The model under review builds one solid part; all positions refer to its coordinate system, in mm. A direction names the side the tool comes from. Round coordinates to 2 decimals unless told otherwise and drop trailing zeros. Order: outer loops, then holes, each group sorted by start corner. A loop starts at its lowest first (then second) coordinate and runs counter-clockwise, first axis right, second up. Notation, with made-up numbers: M 13,57 L 23,57 A12 cw 23,69 Z; hole C 39,-30 d8. An arc over 180 degrees is marked long. Answer as a JSON object with one key per item and string values. Group by question number.
1. To check wall thickness, follow probe 1 along X at (y, z) = (5, 33); probe 2 along X at (y, z) = (7.5, 24.5); probe 3 along X at (y, z) = (-6.5, 54.5). State the ranges of each line that lie inside material, in increasing order. Write a range as [from, to].
2. Add section A-A on y = -5. State the section outline as (x, z) points.
3. Add section B-B on y = 15.5. State the section outline as (x, z) points.
4. Add section C-C on x = 26. State the section outline as (y, z) points.
5. Clearance check with flat-ended pins moving along their axes: P1, Ø2, axis at x = 23, z = 47.5, coming from the +Y side; P2, Ø6.5, axis at x = 20, y = 14, coming from the +Z side; P3, Ø5, axis at y = 21, z = 46, coming from the +X side. State where each tip first meets the part, or that it passes through.
6. Machinability: for faces 1 (the face through (61, 4.572, 28)), 2 (the face through (5.296, 5.336, 45.109)), 3 (the face through (110.308, -5.968, 50.992)), 4 (the face through (5.296, 5.336, 11.708)), which of the approach directions +Z, -Z, +X, -X, +Y, -Y give a long, thin tool a straight path to every point of the face, cutting with its end or side? Answer none if there is none.
7. Add section D-D on z = 35. Give the number of separate pieces and of enclosed holes in the cut face, and give its area (3 significant figures).
8. Mouldability with a two-part tool opening along X and no side actions: class faces 5 (the face through (112.562, -2, 28)), 6 (the face through (0, 16, 28)), 7 (the face through (52, 3, 57.15)), 8 (the face through (71.464, 7.425, 30.463)) as released by +X, released by -X, zero draft, split by the parting line, or undercut.
```python
from build123d import *

# Parameters (mm, degrees)
EXTRUDE1_DEPTH = 57.15
SKETCH2_R      = 14.506414019
EXTRUDE2_DEPTH = 3.175
FILLET1_R      = 2.54
SKETCH3_R      = 11.421445599
EXTRUDE3_DEPTH = 15.875
EXTRUDE4_DEPTH = 2.286
FILLET4_R      = 2.54
FILLET5_R      = 6.35
EXTRUDE5_DEPTH = 4.572
SKETCH6_R      = 4.134080516
EXTRUDE6_DEPTH = 4.572


with BuildPart() as part:
    # Sketch1 → Extrude1 (new body)
    with BuildSketch(Plane.XY):
        Polygon((0, 30.576970443), (0, 0), (107.990032379, 0), (107.990032379, -12.496674877), (112.562032379, -12.496674877), (112.562032379, 4.572), (4.572, 4.572), (4.572, 30.576970443), align=None)
    extrude(amount=EXTRUDE1_DEPTH)

    # Sketch2 → Extrude2 (add)
    with BuildSketch(Plane(origin=(0, 4.572, 0), x_dir=(-1, 0, 0), z_dir=(0, 1, 0))):
        with Locations(Location((-85.846627335, 28.575, 0), (0, 0, 270))):
            Circle(SKETCH2_R)
    extrude(amount=EXTRUDE2_DEPTH)

    # Fillet1
    fillet1_edges = [part.edges().sort_by_distance(p)[0] for p in [
        (85.846627335, 4.572, 43.081414019),
    ]]
    fillet(fillet1_edges, radius=FILLET1_R)

    # Sketch3 → Extrude3 (cut)
    with BuildSketch(Plane(origin=(0, 7.747, 0), x_dir=(-1, 0, 0), z_dir=(0, 1, 0))):
        with Locations(Location((-85.846627335, 28.575, 0), (0, 0, 90))):
            Circle(SKETCH3_R)
    extrude(amount=-EXTRUDE3_DEPTH, mode=Mode.SUBTRACT)

    # Sketch4 → Extrude4 (add, symmetric)
    with BuildSketch(Plane.XY.offset(28.575)):
        Polygon((4.572, 30.576970443), (50.451305306, 4.572), (4.572, 4.572), align=None)
    extrude(amount=EXTRUDE4_DEPTH, both=True)

    # Fillet4
    fillet4_edges = [part.edges().sort_by_distance(p)[0] for p in [
        (27.511652653, 4.572, 26.289),
    ]]
    fillet(fillet4_edges, radius=FILLET4_R)
    fillet4_2_edges = [part.edges().sort_by_distance(p)[0] for p in [
        (27.511652653, 4.572, 30.861),
    ]]
    fillet(fillet4_2_edges, radius=FILLET4_R)
    fillet4_3_edges = [part.edges().sort_by_distance(p)[0] for p in [
        (50.451305306, 4.572, 28.575),
    ]]
    fillet(fillet4_3_edges, radius=FILLET4_R)
    # the kernel refuses this fillet: 2.54 mm, written as the material it adds along each edge
    with BuildSketch(Plane(origin=(4.572, 4.572, 0), x_dir=(1, 0, 0), z_dir=(0, 0, 1))) as fillet4_4_piece_1:
        with BuildLine():
            CenterArc((FILLET4_R, FILLET4_R), FILLET4_R, 180, 90)
            Line((0, FILLET4_R), (-FILLET4_R * 0.02, FILLET4_R))
            Line((-FILLET4_R * 0.02, FILLET4_R), (-FILLET4_R * 0.02, -FILLET4_R * 0.02))
            Line((-FILLET4_R * 0.02, -FILLET4_R * 0.02), (FILLET4_R, -FILLET4_R * 0.02))
            Line((FILLET4_R, -FILLET4_R * 0.02), (FILLET4_R, 0))
        make_face()
    extrude(amount=23.749)
    with BuildSketch(Plane(origin=(4.572, 7.112, 23.749), x_dir=(0, -1, 0), z_dir=(0, 0, -1))) as fillet4_4_piece_2:
        with BuildLine():
            CenterArc((2.54 - FILLET4_R, -FILLET4_R), FILLET4_R, 0, 90)
            Line((2.54 - FILLET4_R, 0), (2.54 - FILLET4_R, FILLET4_R * 0.02))
            Line((2.54 - FILLET4_R, FILLET4_R * 0.02), (2.54, FILLET4_R * 0.02))
            Line((2.54, FILLET4_R * 0.02), (2.54 + FILLET4_R * 0.02, 0))
            Line((2.54 + FILLET4_R * 0.02, 0), (2.54 + FILLET4_R * 0.02, -FILLET4_R))
            Line((2.54 + FILLET4_R * 0.02, -FILLET4_R), (2.54, -FILLET4_R))
        make_face()
    revolve(axis=Axis((4.572, 7.112, 23.749), (-1, 0, 0)), revolution_arc=90)
    with BuildSketch(Plane(origin=(4.572, 7.112, 26.289), x_dir=(0, 0, -1), z_dir=(0, 1, 0))) as fillet4_4_piece_3_section:
        with BuildLine():
            CenterArc((FILLET4_R, -FILLET4_R), FILLET4_R, 90, 90)
            Line((0, -FILLET4_R), (-FILLET4_R * 0.02, -FILLET4_R))
            Line((-FILLET4_R * 0.02, -FILLET4_R), (-FILLET4_R * 0.02, FILLET4_R * 0.02))
            Line((-FILLET4_R * 0.02, FILLET4_R * 0.02), (FILLET4_R, FILLET4_R * 0.02))
            Line((FILLET4_R, FILLET4_R * 0.02), (FILLET4_R, 0))
        make_face()
    fillet4_4_piece_3 = extrude(amount=23.464970443, mode=Mode.PRIVATE)
    fillet4_4_piece_3 = split(fillet4_4_piece_3, bisect_by=Plane(origin=(10.10405857, 27.441329687, 25.709650316), z_dir=(-0.49310869822243814, -0.8699677072957206, 0)), keep=Keep.TOP, mode=Mode.PRIVATE)
    add(fillet4_4_piece_3)
    # the kernel refuses this fillet: 2.54 mm, written as the material it adds along each edge
    with BuildSketch(Plane(origin=(4.572, 4.572, 33.401), x_dir=(1, 0, 0), z_dir=(0, 0, 1))) as fillet4_5_piece_1:
        with BuildLine():
            CenterArc((FILLET4_R, FILLET4_R), FILLET4_R, 180, 90)
            Line((0, FILLET4_R), (-FILLET4_R * 0.02, FILLET4_R))
            Line((-FILLET4_R * 0.02, FILLET4_R), (-FILLET4_R * 0.02, -FILLET4_R * 0.02))
            Line((-FILLET4_R * 0.02, -FILLET4_R * 0.02), (FILLET4_R, -FILLET4_R * 0.02))
            Line((FILLET4_R, -FILLET4_R * 0.02), (FILLET4_R, 0))
        make_face()
    extrude(amount=23.749)
    with BuildSketch(Plane(origin=(4.572, 7.112, 33.401), x_dir=(0, -1, 0), z_dir=(0, 0, 1))) as fillet4_5_piece_2:
        with BuildLine():
            CenterArc((2.54 - FILLET4_R, FILLET4_R), FILLET4_R, 270, 90)
            Line((2.54 - FILLET4_R, 0), (2.54 - FILLET4_R, -FILLET4_R * 0.02))
            Line((2.54 - FILLET4_R, -FILLET4_R * 0.02), (2.54, -FILLET4_R * 0.02))
            Line((2.54, -FILLET4_R * 0.02), (2.54 + FILLET4_R * 0.02, 0))
            Line((2.54 + FILLET4_R * 0.02, 0), (2.54 + FILLET4_R * 0.02, FILLET4_R))
            Line((2.54 + FILLET4_R * 0.02, FILLET4_R), (2.54, FILLET4_R))
        make_face()
    revolve(axis=Axis((4.572, 7.112, 33.401), (1, 0, 0)), revolution_arc=90)
    with BuildSketch(Plane(origin=(4.572, 7.112, 30.861), x_dir=(1, 0, 0), z_dir=(0, 1, 0))) as fillet4_5_piece_3_section:
        with BuildLine():
            CenterArc((FILLET4_R, -FILLET4_R), FILLET4_R, 90, 90)
            Line((0, -FILLET4_R), (-FILLET4_R * 0.02, -FILLET4_R))
            Line((-FILLET4_R * 0.02, -FILLET4_R), (-FILLET4_R * 0.02, FILLET4_R * 0.02))
            Line((-FILLET4_R * 0.02, FILLET4_R * 0.02), (FILLET4_R, FILLET4_R * 0.02))
            Line((FILLET4_R, FILLET4_R * 0.02), (FILLET4_R, 0))
        make_face()
    fillet4_5_piece_3 = extrude(amount=23.464970443, mode=Mode.PRIVATE)
    fillet4_5_piece_3 = split(fillet4_5_piece_3, bisect_by=Plane(origin=(10.10405857, 27.441329687, 31.440349684), z_dir=(-0.49310869822243814, -0.8699677072957206, 0)), keep=Keep.TOP, mode=Mode.PRIVATE)
    add(fillet4_5_piece_3)

    # Fillet5
    fillet5_edges = [part.edges().sort_by_distance(p)[0] for p in [
        (2.286, 30.576970443, 0),
        (110.276032379, -12.496674877, 57.15),
        (2.286, 30.576970443, 57.15),
        (110.276032379, -12.496674877, 0),
    ]]
    fillet(fillet5_edges, radius=FILLET5_R)

    # Sketch5 → Extrude5 (cut)
    with BuildSketch(Plane(origin=(112.562032379, 0, 0), x_dir=(0, 0, -1), z_dir=(1, 0, 0))):
        with BuildLine():
            Line((-48.21617711, -3.129971145), (-8.93382289, -3.129971145))
            ThreePointArc((-8.93382289, -3.129971145), (-6.157220398, -5.906573636), (-8.93382289, -8.683176127))
            Line((-8.93382289, -8.683176127), (-48.21617711, -8.683176127))
            ThreePointArc((-48.21617711, -8.683176127), (-50.992779602, -5.906573636), (-48.21617711, -3.129971145))
        make_face()
    extrude(amount=-EXTRUDE5_DEPTH, mode=Mode.SUBTRACT)

    # Sketch6 → Extrude6 (cut)
    with BuildSketch(Plane(origin=(4.572, 0, 0), x_dir=(0, 0, -1), z_dir=(1, 0, 0))):
        with Locations((-46.51308259, 18.4320182)):
            Circle(SKETCH6_R)
        with Locations(Location((-10.63691741, 18.4320182, 0), (0, 0, 180))):
            Circle(SKETCH6_R)
    extrude(amount=-EXTRUDE6_DEPTH, mode=Mode.SUBTRACT)


solid = part.part
```
Recorded:
{
 "1": {"probe 1": "x = [0, 5.76], [70.85, 75.32], [96.38, 100.84]", "probe 2": "x = [0, 4.69], [71.92, 75.18], [96.52, 99.77]", "probe 3": "x = [107.99, 112.56]"},
 "2": {"outline": "M 107.99,0 L 112.56,0 L 112.56,6.31 L 107.99,6.31 Z; M 107.99,50.84 L 112.56,50.84 L 112.56,57.15 L 107.99,57.15 Z"},
 "3": {"outline": "M 0,0 L 4.57,0 L 4.57,7.72 L 0,7.72 Z; M 0,13.55 L 4.57,13.55 L 4.57,23.75 A2.54 cw 7.11,26.29 L 31.17,26.29 L 31.17,30.86 L 7.11,30.86 A2.54 cw 4.57,33.4 L 4.57,43.6 L 0,43.6 Z; M 0,49.43 L 4.57,49.43 L 4.57,57.15 L 0,57.15 Z"},
 "4": {"outline": "M 0,0 L 4.57,0 L 4.57,23.75 A2.54 cw 7.11,26.29 L 18.43,26.29 L 18.43,30.86 L 7.11,30.86 A2.54 cw 4.57,33.4 L 4.57,57.15 L 0,57.15 Z"},
 "5": {"P1": "stops at y = 4.57", "P2": "stops at z = 30.86", "P3": "stops at x = 4.57"},
 "6": {"face 1": "+Y", "face 2": "+Z, +Y", "face 3": "+X, -X", "face 4": "-Z, +Y"},
 "7": {"separate pieces": "3", "enclosed holes": "0", "area": "606 mm²"},
 "8": {"face 5": "released by +X", "face 6": "released by -X", "face 7": "zero draft", "face 8": "undercut"}
}
